The model under review builds one solid part; all positions refer to its coordinate system, in mm. A direction names the side the tool comes from. Round coordinates to 2 decimals unless told otherwise and drop trailing zeros. Order: outer loops, then holes, each group sorted by start corner. A loop starts at its lowest first (then second) coordinate and runs counter-clockwise, first axis right, second up. Notation, with made-up numbers: (34, 23) -> (66, 23) arc R32 ccw to (66, 51) -> close; hole circle Ø5 at (61.25, 18). An arc over 180 degrees is marked (long way). Put each result on its own line as item: value. Start each with the question number.
from build123d import *

# Parameters (mm, degrees)
SKETCH1_R           = 6.5
SKETCH1_R_2         = 2.5
BOSS_EXTRUDE1_DEPTH = 16
SKETCH2_W           = 1
SKETCH2_H           = 8
SKETCH3_R           = 1.5
CUT_EXTRUDE1_DEPTH  = 7.5
CIRPATTERN1_COUNT   = 2
CIRPATTERN1_ANGLE   = 90
SKETCH6_W           = 0.7
SKETCH6_H           = 8
CUT_EXTRUDE2_DEPTH  = 0.5
CIRPATTERN2_COUNT   = 20


with BuildPart() as part:
    # Sketch1 → Boss-Extrude1 (new body)
    with BuildSketch(Plane(origin=(0, 0, 0), x_dir=(1, 0, 0), z_dir=(0, 1, 0))):
        Circle(SKETCH1_R)
        Circle(SKETCH1_R_2, mode=Mode.SUBTRACT)
    extrude(amount=BOSS_EXTRUDE1_DEPTH)

    # Sketch2 → Cut-Revolve1 (revolve, cut)
    with BuildSketch(Plane.XY):
        with Locations((6, 11)):
            Rectangle(SKETCH2_W, SKETCH2_H)
    revolve(axis=Axis((0, 18.194841433, 0), (0, -1, 0)), mode=Mode.SUBTRACT)

    # Sketch3 → Cut-Extrude1 (cut, through all)
    with BuildSketch(Plane.XY):
        with Locations((0, 3.5)):
            Circle(SKETCH3_R)
    cut_extrude1 = extrude(amount=-CUT_EXTRUDE1_DEPTH, mode=Mode.SUBTRACT)

    # CirPattern1: Cut-Extrude1 ×2 about axis
    cirpattern1_axis = Axis((0, 16, 0), (0, 1, 0))
    for i in range(1, CIRPATTERN1_COUNT):
        add(cut_extrude1.rotate(cirpattern1_axis, i * CIRPATTERN1_ANGLE / (CIRPATTERN1_COUNT - 1)), mode=Mode.SUBTRACT)

    # Sketch6 → Cut-Extrude2 (cut)
    with BuildSketch(Plane.XY.offset(5.5)):
        with Locations((0, 11)):
            Rectangle(SKETCH6_W, SKETCH6_H)
    cut_extrude2 = extrude(amount=-CUT_EXTRUDE2_DEPTH, mode=Mode.SUBTRACT)

    # CirPattern2: Cut-Extrude2 ×20 about axis
    cirpattern2_axis = Axis((0, 0, 0), (0, 1, 0))
    for i in range(1, CIRPATTERN2_COUNT):
        add(cut_extrude2.rotate(cirpattern2_axis, i * 360 / CIRPATTERN2_COUNT), mode=Mode.SUBTRACT)


solid = part.part
Q1. Take a section at C-C on y = 3.5. Give the boundary of the cut face in (x, z).
Q2. Take a section at B-B on z = 0. Give the boundary of the cut face in (x, y), and give its area (3 significant figures).
Q3. Take a section at A-A on x = 0. Give the boundary of the cut face in (y, z).
Q4. Clearance check with flat-ended pins moving along their axes: pin 1 Ø0.8 at (x, y) = (0, 11) entering from +Z; pin 2 Ø2 at (y, z) = (10.5, -0.5) entering from -X; pin 3 Ø2 at (y, z) = (7.5, -2.5) entering from -X. State where each tip first meets the part, or that it passes through.
Q5. For faces 4 (the face through (4.9, 11.1, -2.5)), 5 (the face through (-0.853, 11.056, 5.433)), 6 (the face through (-4.22, 2.17, -0.69)), 7 (the face through (-5.433, 11.056, -0.853)), list the 3-axis set-ups (+Z, -Z, +X, -X, +Y, -Y) from which the entire face can be reached by the end or side of a thin tool; tool diameter is ignored.
Q6. Wall thickness on probe 1 along Y at (x, z) = (0, -5.5); probe 2 along Y at (x, z) = (-3.85, 0); probe 3 along X at (y, z) = (5.75, 0): over which ranges is each line inside the solid? List them lowest first. Write a range as [from, to].
Q7. Draft analysis for pull direction X (two halves, no side actions). For faces 1 (the face through (-2.5, 11.1, 4.9)), 2 (the face through (2.5, 11.1, 4.9)), 3 (the face through (0, 2, -4)), state which applies: +X half, -X half, draft (parallel to the pull), parting line (faces both ways), or undercut.
Calculated:
1. outline: (-6.32, -1.5) arc R6.5 ccw to (-1.5, -6.32) -> (-1.5, -2) arc R2.5 cw to (-2, -1.5) -> close; (-6.32, 1.5) -> (-2, 1.5) arc R2.5 cw (long way) to (1.5, -2) -> (1.5, -6.32) arc R6.5 ccw (long way) to start
2. outline: (-6.5, 0) -> (-2.5, 0) -> (-2.5, 2) -> (-6.5, 2) -> close; (-6.5, 5) -> (-2.5, 5) -> (-2.5, 16) -> (-6.5, 16) -> (-6.5, 15) -> (-5, 15) -> (-5, 7) -> (-6.5, 7) -> close; (2.5, 0) -> (6.5, 0) -> (6.5, 7) -> (5, 7) -> (5, 15) -> (6.5, 15) -> (6.5, 16) -> (2.5, 16) -> close
2. area: 92.0 mm²
3. outline: (0, -6.5) -> (2, -6.5) -> (2, -2.5) -> (0, -2.5) -> close; (0, 2.5) -> (16, 2.5) -> (16, 6.5) -> (15, 6.5) -> (15, 5) -> (7, 5) -> (7, 6.5) -> (0, 6.5) -> close; (5, -6.5) -> (7, -6.5) -> (7, -5) -> (15, -5) -> (15, -6.5) -> (16, -6.5) -> (16, -2.5) -> (5, -2.5) -> close
4. pin 1: stops at z = 5.49
4. pin 2: stops at x = -5.49
4. pin 3: stops at x = -6.29
5. face 4: -Z, +X
5. face 5: +Z, -X
5. face 6: -X
5. face 7: -Z, -X
6. probe 1: y = [0, 2], [5, 7], [15, 16]
6. probe 2: y = [0, 2], [5, 16]
6. probe 3: x = [-6.5, -2.5], [2.5, 6.5]
7. face 1: -X half
7. face 2: +X half
7. face 3: undercut
